from build123d import *

# Parameters (mm, degrees)
SKETCH1_W           = 80
SKETCH1_H           = 30
BOSS_EXTRUDE1_DEPTH = 5
SKETCH2_W           = 20
SKETCH2_H           = 25
CUT_EXTRUDE1_DEPTH  = 86.586213843
BOSS_EXTRUDE2_DEPTH = 35
SKETCH4_R           = 5.5
SKETCH4_R_2         = 1.8
CUT_EXTRUDE2_DEPTH  = 93.330926563
CHAMFER1_SIZE       = 38
CHAMFER1_SIZE2      = 10
FILLET1_R           = 3
SKETCH5_R           = 2.1
CUT_EXTRUDE3_DEPTH  = 95.339811321
SKETCH6_R           = 5
CUT_EXTRUDE4_DEPTH  = 2.4
CHAMFER2_SIZE       = 35
CHAMFER2_SIZE2      = 30
FILLET2_R           = 3
SKETCH7_W           = 6
SKETCH7_H           = 3
SKETCH7_W_2         = 3
SKETCH7_H_2         = 6
BOSS_EXTRUDE3_DEPTH = 40
CHAMFER3_SIZE       = 35
CHAMFER3_SIZE2      = 12
FILLET3_R           = 3
CHAMFER4_SIZE       = 35
CHAMFER4_SIZE2      = 12
FILLET4_R           = 3
SKETCH8_R           = 1.8
CUT_EXTRUDE5_DEPTH  = 95.339811321
CUT_EXTRUDE6_DEPTH  = 93.330926563
FILLET5_R           = 2
CUT_EXTRUDE7_DEPTH  = 3


with BuildPart() as part:
    # Sketch1 → Boss-Extrude1 (new body)
    with BuildSketch(Plane(origin=(0, 0, 0), x_dir=(1, 0, 0), z_dir=(0, 1, 0))):
        with Locations((-40, 15)):
            Rectangle(SKETCH1_W, SKETCH1_H)
    extrude(amount=BOSS_EXTRUDE1_DEPTH)

    # Sketch2 → Cut-Extrude1 (cut, through all)
    with BuildSketch(Plane(origin=(0, 5, 0), x_dir=(1, 0, 0), z_dir=(0, 1, 0))):
        with Locations((-50, 12.5)):
            Rectangle(SKETCH2_W, SKETCH2_H)
    extrude(amount=-CUT_EXTRUDE1_DEPTH, mode=Mode.SUBTRACT)

    # Sketch3 → Boss-Extrude2 (add)
    with BuildSketch(Plane(origin=(0, 5, 0), x_dir=(1, 0, 0), z_dir=(0, 1, 0))):
        Polygon((-80, 30), (0, 30), (0, 25), (-38, 25), (-38, 0), (-40, 0), (-40, 25), (-80, 25), align=None)
    extrude(amount=BOSS_EXTRUDE2_DEPTH)

    # Sketch4 → Cut-Extrude2 (cut, through all)
    with BuildSketch(Plane(origin=(0, 5, 0), x_dir=(1, 0, 0), z_dir=(0, 1, 0))):
        with Locations(Location((-19, 15, 0), (0, 0, 270))):
            Circle(SKETCH4_R)
        with Locations(Location((-7, 15, 0), (0, 0, 270))):
            Circle(SKETCH4_R_2)
        with Locations(Location((-31, 15, 0), (0, 0, 270))):
            Circle(SKETCH4_R_2)
    extrude(amount=-CUT_EXTRUDE2_DEPTH, mode=Mode.SUBTRACT)

    # Chamfer1
    chamfer1_edges = [part.edges().sort_by_distance(p)[0] for p in [
        (0, 2.5, 0),
    ]]
    chamfer1_side = [part.faces().sort_by_distance(p)[0] for p in [
        (-20, 0.565685425, 0),
    ]]
    chamfer(chamfer1_edges, length=CHAMFER1_SIZE, length2=CHAMFER1_SIZE2, reference=chamfer1_side[0])

    # Fillet1
    fillet1_edges = [part.edges().sort_by_distance(p)[0] for p in [
        (0, 2.5, -10),
    ]]
    fillet(fillet1_edges, radius=FILLET1_R)

    # Sketch5 → Cut-Extrude3 (cut, through all)
    with BuildSketch(Plane(origin=(0, 0, -30), x_dir=(-1, 0, 0), z_dir=(0, 0, -1))):
        with Locations((33, 22)):
            Circle(SKETCH5_R)
        with Locations((65, 22)):
            Circle(SKETCH5_R)
    extrude(amount=-CUT_EXTRUDE3_DEPTH, mode=Mode.SUBTRACT)

    # Sketch6 → Cut-Extrude4 (cut)
    with BuildSketch(Plane.XY.offset(-25)):
        with Locations((-33, 22)):
            Circle(SKETCH6_R)
        with Locations((-65, 22)):
            Circle(SKETCH6_R)
    extrude(amount=-CUT_EXTRUDE4_DEPTH, mode=Mode.SUBTRACT)

    # Chamfer2
    chamfer2_edges = [part.edges().sort_by_distance(p)[0] for p in [
        (0, 40, -27.5),
    ]]
    chamfer2_side = [part.faces().sort_by_distance(p)[0] for p in [
        (0, 15.78592553, -25.370407315),
    ]]
    chamfer(chamfer2_edges, length=CHAMFER2_SIZE, length2=CHAMFER2_SIZE2, reference=chamfer2_side[0])

    # Fillet2
    fillet2_edges = [part.edges().sort_by_distance(p)[0] for p in [
        (-30, 40, -27.5),
    ]]
    fillet(fillet2_edges, radius=FILLET2_R)

    # Sketch7 → Boss-Extrude3 (add)
    with BuildSketch(Plane.XZ):
        with Locations((-50, -23.5)):
            Rectangle(SKETCH7_W, SKETCH7_H)
        with Locations((-41.5, -15)):
            Rectangle(SKETCH7_W_2, SKETCH7_H_2)
    extrude(amount=-BOSS_EXTRUDE3_DEPTH)

    # Chamfer3
    chamfer3_edges = [part.edges().sort_by_distance(p)[0] for p in [
        (-39, 40, 0),
    ]]
    chamfer3_side = [part.faces().sort_by_distance(p)[0] for p in [
        (-39, 20, 0),
    ]]
    chamfer(chamfer3_edges, length=CHAMFER3_SIZE, length2=CHAMFER3_SIZE2, reference=chamfer3_side[0])

    # Fillet3
    # the kernel refuses this fillet: 3 mm, written as the material it takes off along each edge
    with BuildSketch(Plane(origin=(-36.75, 5, 0), x_dir=(0, 0.945945945945946, -0.3243243243243238), z_dir=(-1, 0, 0))) as fillet3_piece_1:
        with BuildLine():
            CenterArc((FILLET3_R * 0.166666666667, FILLET3_R), FILLET3_R, 251.075355584, 18.924644416)
            Line((-FILLET3_R * 0.157657657658, FILLET3_R * 0.0540540540541), (0, 0))
            Line((0, 0), (FILLET3_R * 0.166666666667, 0))
        make_face()
    extrude(amount=4.5, mode=Mode.SUBTRACT)
    with BuildSketch(Plane(origin=(-38, -0.970324057, 0), x_dir=(-1, 0, 0), z_dir=(0, 1, 0))) as fillet3_piece_2:
        with BuildLine():
            CenterArc((FILLET3_R * 0.129376540878, -FILLET3_R), FILLET3_R, 90, 14.743562836)
            Line((-FILLET3_R * 0.125116758402, -FILLET3_R * 0.0329254627374), (0, 0))
            Line((0, 0), (FILLET3_R * 0.129376540878, 0))
        make_face()
    extrude(amount=6.940648113, mode=Mode.SUBTRACT)

    # Chamfer4
    chamfer4_edges = [part.edges().sort_by_distance(p)[0] for p in [
        (-80, 40, -27.5),
    ]]
    chamfer4_side = [part.faces().sort_by_distance(p)[0] for p in [
        (-80, 2.5, -0.5),
    ]]
    chamfer(chamfer4_edges, length=CHAMFER4_SIZE, length2=CHAMFER4_SIZE2, reference=chamfer4_side[0])

    # Fillet4
    fillet4_edges = [part.edges().sort_by_distance(p)[0] for p in [
        (-68, 40, -27.5),
    ]]
    fillet(fillet4_edges, radius=FILLET4_R)

    # Sketch8 → Cut-Extrude5 (cut, through all)
    with BuildSketch(Plane.XZ):
        with Locations(Location((-74, -15, 0), (0, 0, 270))):
            Circle(SKETCH8_R)
    extrude(amount=-CUT_EXTRUDE5_DEPTH, mode=Mode.SUBTRACT)

    # Sketch9 → Cut-Extrude6 (cut, through all)
    with BuildSketch(Plane(origin=(0, 5, 0), x_dir=(1, 0, 0), z_dir=(0, 1, 0))):
        Polygon((-80, 10), (-70, 10), (-66, 25), (-60, 25), (-60, 0), (-80, 0), align=None)
    extrude(amount=-CUT_EXTRUDE6_DEPTH, mode=Mode.SUBTRACT)

    # Fillet5
    fillet5_edges = [part.edges().sort_by_distance(p)[0] for p in [
        (-80, 2.5, -10),
        (-70, 2.5, -10),
        (-66, 2.5, -25),
        (-73, 5, -25),
    ]]
    fillet(fillet5_edges, radius=FILLET5_R)

    # Sketch10 → Cut-Extrude7 (cut)
    with BuildSketch(Plane(origin=(0, 5, 0), x_dir=(1, 0, 0), z_dir=(0, 1, 0))):
        Polygon((-71.1, 13.325684219), (-71.1, 16.674315781), (-74, 18.348631561), (-76.9, 16.674315781), (-76.9, 13.325684219), (-74, 11.651368439), align=None)
    extrude(amount=-CUT_EXTRUDE7_DEPTH, mode=Mode.SUBTRACT)


solid = part.part
Work out the finished part from the listing and answer in its coordinate system (mm). A direction names the side the tool comes from. Coordinates: 2 decimals unless noted, no trailing zeros. Order: outer loops, then holes, each group sorted by start corner. A loop starts at its lowest first (then second) coordinate and runs counter-clockwise, first axis right, second up. Notation, with made-up numbers: (51, 37) - (79, 37) arc R8 ccw to (79, 41) - close; hole circle Ø6 at (-31.5, 37). An arc over 180 degrees is marked (long way). Put each result on its own line as item: value. Start each with the question number.
1) For faces 1 (the flat face through (-68.02, 2.57, -17.42)), 2 (the flat face through (-23, 18, -25)), 3 (the cylindrical face through (-37, 19, -26)), 4 (the flat face through (-39, 2, 0)), 5 (the flat face through (-75, 5, -18)), determine the directions among +Z, -Z, +X, -X, +Y, -Y from which every point of the face is accessible in a straight line to the end or side of a thin tool.
2) Find section A-A (x = -7). Give the vertices of the cut face in (y, z).
3) Find section D-D (y = 35.5). Give the vertices of the cut face in (x, z).
4) Flat-ended cylindrical pins translate along their axes: pin 1 (4 mm diameter, centred on x = -69, y = 20, fed in from +Z); pin 2 (12 mm diameter, centred on y = 30.5, z = -25.5, fed in from +X); pin 3 (10.5 mm diameter, centred on x = -75, z = -19, fed in from +Y). Find the tip coordinate at first contact, or state that the pin passes through.
5) For a pull along X with two mould halves and no side action, classify faces 6 (the cylindrical face through (-30.11, 39.72, -27.46)), 7 (the cylindrical face through (-67.58, 39.456, -27.535)), 8 (the cylindrical face through (-29.215, 2.535, -15.234)) as released by +X, released by -X, zero draft, split by the parting line, or undercut.
6) Find the intervals of material crossed by line 1 (Y direction, x = -65, z = -29.1); line 2 (Y direction, x = -33, z = -26.05); line 3 (X direction, y = 21.5, z = -27), in increasing order. Write a range as from..to.
7) Find section B-B (z = -15). State how many separate pieces and enclosed holes the cut face has, plus the area to 3 significant figures.
8) Find section C-C (x = -19). Give the vertices of the cut face in (y, z), plus the area to 3 significant figures.
Results list:
1. face 1: +Z, +Y, -Y
1. face 2: +Z, +X, +Y
1. face 3: +Z
1. face 4: +Z, +X, -X, +Y, -Y
1. face 5: +Z, -X, +Y
2. outline: (0, -30) - (13.17, -30) - (13.17, -25) - (5, -25) - (5, -16.8) - (0, -16.8) - close; (0, -13.2) - (5, -13.2) - (5, -8.16) - (0, -8.16) - close
3. outline: (-69.54, -30) - (-26.14, -30) - (-26.14, -25) - (-38, -25) - (-38, -10.46) - (-40, -10.46) - (-40, -12) - (-43, -12) - (-43, -18) - (-40, -18) - (-40, -25) - (-47, -25) - (-47, -22) - (-53, -22) - (-53, -25) - (-69.54, -25) - close
4. pin 1: stops at z = -25
4. pin 2: stops at x = -16.71
4. pin 3: stops at y = 5.44
5. face 6: released by +X
5. face 7: released by -X
5. face 8: undercut
6. line 1: y = 0..19.9, 24.1..40
6. line 2: y = 0..17, 27..40
6. line 3: x = -74.34..-69.97, -60.03..-37.97, -28.03..-14.14
7. separate pieces: 6
7. enclosed holes: 0
7. area: 331 mm^2
8. outline: (0, -30) - (27.17, -30) - (27.17, -25) - (5, -25) - (5, -20.5) - (0, -20.5) - close; (0, -9.5) - (5, -9.5) - (5, -5) - (0, -5) - close
8. area: 181 mm^2
